For this review, take the finished solid that the model builds, in its own axes (mm). A direction names the side the tool comes from. Give positions to 0.01 mm unless a question says otherwise; leave off trailing zeros. Write each loop counter-clockwise with the first axis right and the second up, starting at its lowest first coordinate (ties: lowest second). Pieces come first, ordered by that corner, then holes. Notation, with made-up numbers: M 46,39.5 L 100,39.5 A25 ccw 100,70.5 Z; hole C 11.25,50 d9. An arc over 180 degrees is marked long. Write item = value, one per line.
```python
from build123d import *

# Parameters (mm, degrees)
SKETCH001_W  = 90
SKETCH001_H  = 45
PAD_DEPTH    = 2.5
SKETCH_R     = 4
SKETCH_R_2   = 1
PAD001_DEPTH = 6.5
FILLET_R     = 6
FILLET001_R  = 1.5


with BuildPart() as part:
    # Sketch001 → Pad (new body)
    with BuildSketch(Plane.XY):
        Rectangle(SKETCH001_W, SKETCH001_H)
    extrude(amount=PAD_DEPTH)

    # Sketch → Pad001 (join)
    with BuildSketch(Plane.XY):
        with Locations((-37.5, 15)):
            Circle(SKETCH_R)
        with Locations((-37.5, 15)):
            Circle(SKETCH_R_2, mode=Mode.SUBTRACT)
        with Locations((37.5, 15)):
            Circle(SKETCH_R)
        with Locations((37.5, 15)):
            Circle(SKETCH_R_2, mode=Mode.SUBTRACT)
        with Locations((37.5, -15)):
            Circle(SKETCH_R)
        with Locations((37.5, -15)):
            Circle(SKETCH_R_2, mode=Mode.SUBTRACT)
        with Locations((-37.5, -15)):
            Circle(SKETCH_R)
        with Locations((-37.5, -15)):
            Circle(SKETCH_R_2, mode=Mode.SUBTRACT)
    extrude(amount=PAD001_DEPTH)

    # Fillet
    fillet_edges = [part.edges().sort_by_distance(p)[0] for p in [
        (45, -22.5, 1.25),
        (45, 22.5, 1.25),
        (-45, 22.5, 1.25),
        (-45, -22.5, 1.25),
    ]]
    fillet(fillet_edges, radius=FILLET_R)

    # Fillet001
    fillet001_edges = [part.edges().sort_by_distance(p)[0] for p in [
        (-45, 0, 2.5),
        (-43.242641, 20.742641, 2.5),
        (-43.242641, -20.742641, 2.5),
        (0, 22.5, 2.5),
        (0, -22.5, 2.5),
        (43.242641, 20.742641, 2.5),
        (43.242641, -20.742641, 2.5),
        (45, 0, 2.5),
        (-41.5, -15, 2.5),
        (33.5, -15, 2.5),
        (-41.5, 15, 2.5),
        (33.5, 15, 2.5),
    ]]
    fillet(fillet001_edges, radius=FILLET001_R)


solid = part.part
```
1. We need section C-C, the plane y = -6.5. Write out the cut boundary in (x, z), then the cut area to 3 significant figures.
Responses:
outline = M -45,0 L 45,0 L 45,1 A1.5 ccw 43.5,2.5 L -43.5,2.5 A1.5 ccw -45,1 Z
area = 224 mm2
2. Machinability: for faces 1 (the face through (43.196, -20.789, 0.507)), 2 (the face through (-37.04, 14.11, 4.47)), which of the approach directions +Z, -Z, +X, -X, +Y, -Y give a long, thin tool a straight path to every point of the face, cutting with its end or side? Answer none if there is none.
Responses:
face_1 = +Z, -Z, +X, -Y
face_2 = +Z
3. Insertion check: P1, Ø6, axis at x = -19.5, y = 15.5, coming from the +Z side; P2, Ø2, axis at x = -19.5, z = 3, coming from the +Y side. Each pin has a flat end and moves straight along its axis. Give the tip position at first contact, or say it passes through.
Responses:
P1 = 2.5
P2 = 22.12
4. The part is to be moulded in two halves that separate along X. For faces 3 (the face through (-1, 0, 0)), 4 (the face through (-37.04, -15.89, 4.47)), 5 (the face through (43.196, 20.789, 0.507)), 6 (the face through (-43.289, 20.696, 0.507)), say which applies: +X half, -X half, draft (parallel to the pull), parting line (faces both ways), or undercut.
Responses:
face_3 = draft
face_4 = undercut
face_5 = +X half
face_6 = -X half
5. For line 1 along Y through (x, z) = (37.5, 5.35); line 2 along X through (y, z) = (-15, 4.35); line 3 along Z through (x, y) = (32, -18.5), list the stretches that pass through material, from the lowest coordinate up. Write a range as from..to.
Responses:
line_1 = -19..-16, -14..-11, 11..14, 16..19
line_2 = -41.5..-38.5, -36.5..-33.5, 33.5..36.5, 38.5..41.5
line_3 = 0..2.5
6. We need section B-B, the plane x = -31. Write out the cut boundary in (y, z), then the cut area to 3 significant figures.
Responses:
outline = M -22.5,0 L 22.5,0 L 22.5,1 A1.5 ccw 21,2.5 L -21,2.5 A1.5 ccw -22.5,1 Z
area = 112 mm2
7. We need section A-A, the plane y = 15. Write out the cut boundary in (x, z), then the cut area to 3 significant figures.
Responses:
outline = M -45,0 L 45,0 L 45,1 A1.5 ccw 43.5,2.5 L 43,2.5 A1.5 cw 41.5,4 L 41.5,6.5 L 38.5,6.5 L 38.5,2.5 L 36.5,2.5 L 36.5,6.5 L 33.5,6.5 L 33.5,4 A1.5 cw 32,2.5 L -32,2.5 A1.5 cw -33.5,4 L -33.5,6.5 L -36.5,6.5 L -36.5,2.5 L -38.5,2.5 L -38.5,6.5 L -41.5,6.5 L -41.5,4 A1.5 cw -43,2.5 L -43.5,2.5 A1.5 ccw -45,1 Z
area = 274 mm2
